The listing builds one solid part. Answer for the finished solid, in the listing's coordinates (mm). A direction names the side the tool comes from. Give positions to 0.01 mm unless a question says otherwise; leave off trailing zeros. Order: outer loops, then holes, each group sorted by start corner. A loop starts at its lowest first (then second) coordinate and runs counter-clockwise, first axis right, second up. Notation, with made-up numbers: M 62,26.5 L 114,26.5 A37 ccw 114,64.5 Z; hole C 61.25,-29.5 d5. An arc over 180 degrees is marked long. Answer as a JSON object with one key per item and string values. Group by question number.
```python
from build123d import *

# Parameters (mm, degrees)
SKETCH1_R                = 15
SKETCH1_R_2              = 7.5
BOSS_EXTRUDE1_DEPTH      = 42
SKETCH2_W                = 46
SKETCH2_H                = 40
BOSS_EXTRUDE2_DEPTH      = 23
SKETCH3_W                = 24
SKETCH3_H                = 30
CUT_EXTRUDE1_DEPTH       = 66.421708935
HOLE1_D                  = 15
BOSS_EXTRUDE3_DEPTH      = 11
BOSS_EXTRUDE3_DEPTH_BACK = 55
SKETCH6_R                = 18
SKETCH7_W                = 24
SKETCH7_H                = 30
CUT_EXTRUDE2_DEPTH       = 72.449282712
HOLE2_D                  = 18


with BuildPart() as part:
    # Sketch1 → Boss-Extrude1 (new, symmetric)
    with BuildSketch(Plane(origin=(0, 0, 0), x_dir=(0, 0, -1), z_dir=(1, 0, 0))):
        with Locations(Location((0, 0, 0), (0, 0, 180))):
            Circle(SKETCH1_R)
        with Locations(Location((0, 0, 0), (0, 0, 180))):
            Circle(SKETCH1_R_2, mode=Mode.SUBTRACT)
    extrude(amount=BOSS_EXTRUDE1_DEPTH, both=True)

    # Sketch2 → Boss-Extrude2 (add, symmetric)
    with BuildSketch(Plane.XY):
        Rectangle(SKETCH2_W, SKETCH2_H)
    extrude(amount=BOSS_EXTRUDE2_DEPTH, both=True)

    # Sketch3 → Cut-Extrude1 (cut, through all)
    with BuildSketch(Plane.XY.offset(23)):
        Rectangle(SKETCH3_W, SKETCH3_H)
    extrude(amount=-CUT_EXTRUDE1_DEPTH, mode=Mode.SUBTRACT)

    # Hole1 (through all)
    with Locations(Plane(origin=(42, 0, 0), x_dir=(0, 0, -1), z_dir=(1, 0, 0))):
        with Locations((0, 0)):
            Hole(HOLE1_D / 2)

    # Sketch6 → Boss-Extrude3 (add, two sides: drawn at the far end of the back side and taken through both)
    with BuildSketch(Plane(origin=(0, 20, 0), x_dir=(1, 0, 0), z_dir=(0, 1, 0)).offset(-BOSS_EXTRUDE3_DEPTH_BACK)):
        with Locations(Location((0, 0, 0), (0, 0, 270))):
            Circle(SKETCH6_R)
    extrude(amount=BOSS_EXTRUDE3_DEPTH + BOSS_EXTRUDE3_DEPTH_BACK)

    # Sketch7 → Cut-Extrude2 (cut, through all)
    with BuildSketch(Plane.XY.offset(23)):
        Rectangle(SKETCH7_W, SKETCH7_H)
    extrude(amount=-CUT_EXTRUDE2_DEPTH, mode=Mode.SUBTRACT)

    # Hole2 (through all)
    with Locations(Plane(origin=(0, 31, 0), x_dir=(1, 0, 0), z_dir=(0, 1, 0))):
        with Locations((0, 0)):
            Hole(HOLE2_D / 2)


solid = part.part
```
Item 1: Section B-B (y = 0) is taken. Determine the outline of the cut face in (x, z), and give its area (3 significant figures).
Item 2: Flat-ended cylindrical pins translate along their axes: P1, Ø6, axis at x = -23, z = 3, coming from the +Y side; P2, Ø3, axis at y = -27.5, z = 0, coming from the -X side; P3, Ø5, axis at x = 27.5, y = -2.5, coming from the +Z side. Find the tip coordinate at first contact, or state that the pin passes through.
Item 3: Section D-D (y = 26) is taken. Determine the outline of the cut face in (x, z).
Item 4: Determine the mould class of faces 4 (the flat face through (-42, -7, -4)), 5 (the flat face through (-16, 0, -23)), 6 (the cylindrical face through (1.172, 22.888, -8.923)) for opening direction Z: released by +Z, released by -Z, zero draft, split by the parting line, or undercut.
Item 5: Section C-C (x = -22) is taken. Determine the outline of the cut face in (y, z).
Item 6: Consider probe 1 along Z at (x, y) = (0, -28); probe 2 along X at (y, z) = (-12.5, 17); probe 3 along Y at (x, z) = (-31, 0). Determine where each line is inside the solid, lowest interval first. Write a range as from..to.
Item 7: Section A-A (x = 0) is taken. Determine the outline of the cut face in (y, z).
Item 8: A tool of negligible diameter and unlimited length cuts with its end or side. For faces 1 (the flat face through (-16, -20, 11)), 2 (the flat face through (23, 0, 16)), 3 (the flat face through (-12, 0, 0)), from which of +Z, -Z, +X, -X, +Y, -Y can it reach the whole face along a straight path? Write none if from no direction.
Values found:
{
 "1": {"outline": "M -42,-15 L -23,-15 L -23,-23 L -12,-23 L -12,23 L -23,23 L -23,15 L -42,15 L -42,7.5 L -16.36,7.5 A18 ccw -16.36,-7.5 L -42,-7.5 Z; M 12,-23 L 23,-23 L 23,-15 L 42,-15 L 42,-7.5 L 16.36,-7.5 A18 ccw 16.36,7.5 L 42,7.5 L 42,15 L 23,15 L 23,23 L 12,23 Z", "area": "1,420 mm^2"},
 "2": {"P1": "stops at y = 20", "P2": "stops at x = -18", "P3": "stops at z = 15"},
 "3": {"outline": "C 0,0 d36; hole C 0,0 d18"},
 "4": {"face 4": "zero draft", "face 5": "released by -Z", "face 6": "undercut"},
 "5": {"outline": "M -20,-23 L 20,-23 L 20,23 L -20,23 Z; hole C 0,0 d15"},
 "6": {"probe 1": "z = -18..-9, 9..18", "probe 2": "x = -23..-12, 12..23", "probe 3": "y = -15..-7.5, 7.5..15"},
 "7": {"outline": "M -35,-18 L -20,-18 L -20,-23 L -15,-23 L -15,-9 L -35,-9 Z; M -35,9 L -15,9 L -15,23 L -20,23 L -20,18 L -35,18 Z; M 15,-23 L 20,-23 L 20,-18 L 31,-18 L 31,-9 L 15,-9 Z; M 15,9 L 31,9 L 31,18 L 20,18 L 20,23 L 15,23 Z"},
 "8": {"face 1": "-Y", "face 2": "+X", "face 3": "+Z, -Z"}
}
